```python
from build123d import *
from build123d.topology import SkipClean

# Parameters (mm, degrees)
SKETCH1_W            = 15
SKETCH1_H            = 15
SKETCH1_R            = 1.1
EXTRUDE1_DEPTH       = 4
EXTRUDE2_DEPTH       = 60
EXTRUDE2_DEPTH_BACK  = 4
SKETCH3_R            = 2
SKETCH4_R            = 1.75
EXTRUDE3_DEPTH       = 3
SKETCH5_R            = 2
EXTRUDE4_DEPTH       = 3
SKETCH9_R            = 0.5
EXTRUDE8_DEPTH       = 63
EXTRUDE_START        = 1
SKETCH_4_W           = 15
SKETCH_4_H           = 15
SKETCH_4_R           = 1.1
EXTRUDE_1_DEPTH      = 1
SKETCH_3_R           = 1.5
CUT_EXTRUDE_2_DEPTH  = 104
SKETCH_5_W           = 63.20966087
SKETCH_5_H           = 58.197081521
CUT_EXTRUDE_3_DEPTH  = 40
EXTRUDE_2_DEPTH      = 5
EXTRUDE_2_DEPTH_BACK = 10
SKETCH_6_R           = 2.25
SKETCH_6_R_2         = 1.5
CUT_EXTRUDE_START    = -1.5
SKETCH_7_R           = 2.25
CUT_EXTRUDE_4_DEPTH  = 1.5


with BuildPart() as part:
    # Sketch1 → Extrude1 (new body)
    with BuildSketch(Plane.XY):
        with Locations((7.5, -7.5)):
            Rectangle(SKETCH1_W, SKETCH1_H)
        with Locations((3.5, -3.5)):
            Circle(SKETCH1_R, mode=Mode.SUBTRACT)
        with Locations((11.5, -3.5)):
            Circle(SKETCH1_R, mode=Mode.SUBTRACT)
        with Locations((11.5, -11.5)):
            Circle(SKETCH1_R, mode=Mode.SUBTRACT)
        with Locations((3.5, -11.5)):
            Circle(SKETCH1_R, mode=Mode.SUBTRACT)
    extrude(amount=EXTRUDE1_DEPTH)

    # Sketch3 → Extrude2 (add, two sides: drawn at the far end of the back side and taken through both)
    with BuildSketch(Plane(origin=(0, -5.75, 5.75), x_dir=(1, 0, 0), z_dir=(0, -0.7071067811865488, 0.7071067811865464)).offset(-EXTRUDE2_DEPTH_BACK)):
        with Locations(Location((7.5, -2.474873734, 0), (0, 0, 270))):
            Circle(SKETCH3_R)
    extrude(amount=EXTRUDE2_DEPTH + EXTRUDE2_DEPTH_BACK)

    # Sketch4 → Extrude3 (add)
    with BuildSketch(Plane(origin=(0, -48.176406871, 48.176406871), x_dir=(1, 0, 0), z_dir=(0, -0.7071067811865487, 0.7071067811865465))):
        with Locations(Location((7.5, -2.474873734, 0), (0, 0, 90))):
            Circle(SKETCH4_R)
    extrude(amount=EXTRUDE3_DEPTH)

    # Sketch5 → Extrude4 (add)
    with BuildSketch(Plane(origin=(0, -50.297727215, 50.297727215), x_dir=(-1, 0, 0), z_dir=(0, -0.7071067811865486, 0.7071067811865465))):
        with Locations(Location((-7.5, 2.474873734, 0), (0, 0, 90))):
            Circle(SKETCH5_R)
    extrude(amount=EXTRUDE4_DEPTH)

    # Sketch9 → Extrude8 (cut)
    with BuildSketch(Plane(origin=(0, 0, 0), x_dir=(0, 0, -1), z_dir=(1, 0, 0))):
        with Locations(Location((-47.487067043, -50.987067043, 0), (0, 0, 180))):
            Circle(SKETCH9_R)
    extrude(amount=EXTRUDE8_DEPTH, mode=Mode.SUBTRACT)

    # 草图4 → 凸台-拉伸1 (add)
    with SkipClean():  # the faces are left unmerged after this step: merging them gives an invalid solid
        with BuildSketch(Plane(origin=(0, 0, 0), x_dir=(-1, 0, 0), z_dir=(0, 0, -1)).offset(EXTRUDE_START)):
            with Locations((-7.5, -7.5)):
                Rectangle(SKETCH_4_W, SKETCH_4_H)
            with Locations((-3.5, -3.5)):
                Circle(SKETCH_4_R, mode=Mode.SUBTRACT)
            with Locations((-11.5, -3.5)):
                Circle(SKETCH_4_R, mode=Mode.SUBTRACT)
            with Locations((-11.5, -11.5)):
                Circle(SKETCH_4_R, mode=Mode.SUBTRACT)
            with Locations((-3.5, -11.5)):
                Circle(SKETCH_4_R, mode=Mode.SUBTRACT)
        extrude(amount=-EXTRUDE_1_DEPTH)

    # 草图3 → 切除-拉伸2 (cut)
    with BuildSketch(Plane(origin=(0, -52.419047558, 52.419047558), x_dir=(1, 0, 0), z_dir=(0, -0.7071067811865487, 0.7071067811865465))):
        with Locations(Location((7.5, -2.474873734, 0), (0, 0, 270))):
            Circle(SKETCH_3_R)
    extrude(amount=-CUT_EXTRUDE_2_DEPTH, mode=Mode.SUBTRACT)

    # 草图5 → 切除-拉伸3 (cut)
    with SkipClean():  # the faces are left unmerged after this step: merging them gives an invalid solid
        with BuildSketch(Plane(origin=(15, 0, 0), x_dir=(0, 0, -1), z_dir=(1, 0, 0))):
            with Locations((-35.604830435, -29.098540761)):
                Rectangle(SKETCH_5_W, SKETCH_5_H)
        extrude(amount=-CUT_EXTRUDE_3_DEPTH, mode=Mode.SUBTRACT)
    add(part.part.scale(1), mode=Mode.REPLACE)  # the faces are merged on a copy

    # 草图6 → 凸台-拉伸2 (add, two sides: drawn at the far end of the back side and taken through both)
    with BuildSketch(Plane(origin=(0, -5.75, 5.75), x_dir=(1, 0, 0), z_dir=(0, -0.7071067811865488, 0.7071067811865464)).offset(-EXTRUDE_2_DEPTH_BACK)):
        with Locations(Location((7.5, -2.474873734, 0), (0, 0, 270))):
            Circle(SKETCH_6_R)
        with Locations(Location((7.5, -2.474873734, 0), (0, 0, 270))):
            Circle(SKETCH_6_R_2, mode=Mode.SUBTRACT)
    extrude(amount=EXTRUDE_2_DEPTH + EXTRUDE_2_DEPTH_BACK)

    # 草图7 → 切除-拉伸4 (cut)
    with SkipClean():  # the faces are left unmerged after this step: merging them gives an invalid solid
        with BuildSketch(Plane(origin=(0, 1.321067812, -1.321067812), x_dir=(1, 0, 0), z_dir=(0, 0.7071067811865487, -0.7071067811865465)).offset(CUT_EXTRUDE_START)):
            with Locations(Location((7.5, 2.474873734, 0), (0, 0, 90))):
                Circle(SKETCH_7_R)
        extrude(amount=CUT_EXTRUDE_4_DEPTH, mode=Mode.SUBTRACT)


solid = part.part
```
Input: part model. Units: mm. Frame: model coordinates. Give positions to 0.01 mm unless a question says otherwise; leave off trailing zeros. Order: outer loops, then holes, each group sorted by start corner. A loop starts at its lowest first (then second) coordinate and runs counter-clockwise, first axis right, second up. Notation, with made-up numbers: M -28.5,-36.5 L 4.5,-36.5 A23 cw 4.5,-19.5 Z; hole C -20,9.25 d4. An arc over 180 degrees is marked long. Return JSON: item names as keys, results as strings.
1) Contact query for flat-ended pins moving along their axis: pin 1 (3 mm diameter, centred on x = 11.5, y = -11.5, fed in from -Z); pin 2 (2.5 mm diameter, centred on x = 11.5, y = -3.5, fed in from +Z); pin 3 (2.5 mm diameter, centred on x = 7.5, z = 2, fed in from +Y). Output: stop coordinate, or through.
Taken from the geometry:
{"pin 1": "stops at z = -1", "pin 2": "stops at z = 4", "pin 3": "stops at y = 0"}
2) Section query A-A on x = 11.5. Output: boundary loops of the cut face in (y, z).
Taken from the geometry:
{"outline": "M -15,-1 L -12.6,-1 L -12.6,4 L -15,4 Z; M -10.4,-1 L -4.6,-1 L -4.6,4 L -10.4,4 Z; M -2.4,-1 L 0,-1 L 0,4 L -2.4,4 Z"}
3) Section query B-B on y = -2.75. Count the separate pieces of the cut face and the enclosed holes in it, and give its area (3 significant figures).
Taken from the geometry:
{"separate pieces": "3", "enclosed holes": "1", "area": "57.8 mm2"}
4) Section query D-D on y = -13.25. Output: boundary loops of the cut face in (x, z), and give its area (3 significant figures).
Taken from the geometry:
{"outline": "M 0,-1 L 15,-1 L 15,4 L 0,4 Z", "area": "75.0 mm2"}
5) Mould query, pull axis Z, two halves, no side actions, for faces 1 (the face through (6.036, -5.966, 2.926)), 2 (the face through (8, 0, 1)). Classes: released by +Z, released by -Z, zero draft, split by the parting line, or undercut.
Taken from the geometry:
{"face 1": "undercut", "face 2": "zero draft"}
6) Line query: L1, parallel to Y at x = 11.5, z = 2; L2, parallel to X at y = -3.5, z = 2.7; L3, parallel to X at y = -3.5, z = -0.6. Output: solid intervals per line, ascending. Write a range as [from, to].
Taken from the geometry:
{"L1": "y = [-15, -12.6], [-10.4, -4.6], [-2.4, 0]", "L2": "x = [0, 2.4], [4.6, 10.4], [12.6, 15]", "L3": "x = [0, 2.4], [4.6, 6.06], [8.94, 10.4], [12.6, 15]"}
7) Section query C-C on x = 7.75. Output: boundary loops of the cut face in (y, z), and give its area (3 significant figures).
Taken from the geometry:
{"outline": "M -15,-1 L -5.66,-1 L -3.07,-3.59 L -2.54,-3.06 L -12.08,6.49 L -12.62,5.95 L -10.66,4 L -15,4 Z; M -9.99,8.58 L -0.44,-0.96 L 0.09,-0.43 L 0,-0.34 L 0,4 L -4.34,4 L -9.45,9.12 Z", "area": "64.0 mm2"}
